```python
from build123d import *

# Parameters (mm, degrees)
F1_DEPTH  = 200
F2_R      = 15.75
F2_R_2    = 8.75
F3_DEPTH  = 20
F4_DEPTH  = 40.001
F6_DEPTH  = 89
F5_R      = 50
F7_DEPTH  = 221
F8_D      = 12.1
F9_W      = 50
F9_H      = 60
F10_DEPTH = 50
F12_DEPTH = 125.001
F13_R     = 10
F14_SIZE  = 10
F15_SIZE  = 5
F16_SIZE  = 10
F20_D     = 12.1


with BuildPart() as f1:
    # F0 (on Front) → F1 (new body)
    with BuildSketch(Plane.XZ):
        Polygon((-300, 0), (0, 0), (0, 40), (-260, 40), (-260, 300), (-300, 300), align=None)
    extrude(amount=-F1_DEPTH)

    # F2 (on face) → F3 (cut)
    with BuildSketch(Plane.XY.offset(40)):
        with Locations((-160, 160)):
            Circle(F2_R)
        with Locations((-160, 160)):
            Circle(F2_R_2, mode=Mode.SUBTRACT)
        with Locations((-160, 40)):
            Circle(F2_R)
        with Locations((-160, 40)):
            Circle(F2_R_2, mode=Mode.SUBTRACT)
        with BuildLine():
            ThreePointArc((-24.25, 40), (-28.8630681963, 51.1369318037), (-40, 55.75))
            ThreePointArc((-40, 55.75), (-51.1369318037, 28.8630681963), (-24.25, 40))
        make_face()
        with BuildLine():
            ThreePointArc((-31.25, 40), (-46.1871843354, 33.8128156646), (-40, 48.75))
            ThreePointArc((-40, 48.75), (-33.8128156646, 46.1871843354), (-31.25, 40))
        make_face(mode=Mode.SUBTRACT)
        with BuildLine():
            ThreePointArc((-24.25, 160), (-51.1369318037, 171.1369318037), (-40, 144.25))
            ThreePointArc((-40, 144.25), (-28.8630681963, 148.8630681963), (-24.25, 160))
        make_face()
        with BuildLine():
            ThreePointArc((-31.25, 160), (-33.8128156646, 153.8128156646), (-40, 151.25))
            ThreePointArc((-40, 151.25), (-46.1871843354, 166.1871843354), (-31.25, 160))
        make_face(mode=Mode.SUBTRACT)
    extrude(amount=-F3_DEPTH, mode=Mode.SUBTRACT)

    # F4 (cut, through all): faces of the model
    f4_faces = [f1.faces().sort_by_distance(p)[0] for p in [
        (-160, 160, 40),
        (-40, 160, 40),
        (-40, 40, 40),
        (-160, 40, 40),
    ]]
    extrude(f4_faces, amount=-F4_DEPTH, mode=Mode.SUBTRACT)

    # F5 (on face) → F6 (cut)
    with BuildSketch(Plane.YZ.offset(-260)):
        with BuildLine():
            ThreePointArc((0, 200), (29.2893218813, 270.7106781187), (100, 300))
            Line((100, 300), (0, 300))
            Line((0, 300), (0, 200))
        make_face()
        with BuildLine():
            ThreePointArc((100, 300), (170.7106781187, 270.7106781187), (200, 200))
            Line((200, 200), (200, 300))
            Line((200, 300), (100, 300))
        make_face()
    extrude(amount=-F6_DEPTH, mode=Mode.SUBTRACT)

    # F5 (on face) → F7 (cut)
    with BuildSketch(Plane.YZ.offset(-260)):
        with Locations((100, 200)):
            Circle(F5_R)
    extrude(amount=-F7_DEPTH, mode=Mode.SUBTRACT)

    # F8 (through all)
    with Locations(Plane.YZ.offset(-260)):
        with Locations((28, 200), (100, 272), (172, 200), (100, 128)):
            Hole(F8_D / 2)

    # F9 (on face) → F10 (join)
    with BuildSketch(Plane.YZ.offset(-260)):
        with Locations((100, 70)):
            Rectangle(F9_W, F9_H)
    extrude(amount=F10_DEPTH)

    # F11 (on face) → F12 (cut, through all)
    with BuildSketch(Plane.XZ.offset(-75)):
        Polygon((-210, 100), (-260, 100), (-210, 40), align=None)
    extrude(amount=-F12_DEPTH, mode=Mode.SUBTRACT)

    # F13
    f13_edges = [f1.edges().sort_by_distance(p)[0] for p in [
        (-260, 37.5, 40),
        (-260, 162.5, 40),
    ]]
    fillet(f13_edges, radius=F13_R)

    # F14
    f14_edges = [f1.edges().sort_by_distance(p)[0] for p in [
        (0, 0, 20),
        (0, 200, 20),
    ]]
    chamfer(f14_edges, length=F14_SIZE)

    # F15
    f15_edges = [f1.edges().sort_by_distance(p)[0] for p in [
        (-260, 50, 200),
        (-300, 50, 200),
    ]]
    chamfer(f15_edges, length=F15_SIZE)

    # F16
    f16_edges = [f1.edges().sort_by_distance(p)[0] for p in [
        (-300, 100, 0),
    ]]
    chamfer(f16_edges, length=F16_SIZE)

    # F20 (through all)
    with Locations(Plane(origin=(0, -120.7106781187, 120.7106781187), x_dir=(1, 0, 0), z_dir=(0, -0.7071067812, 0.7071067812))):
        with Locations((-280, 212.132034356)):
            Hole(F20_D / 2)


solid = f1.part
```
Verification items for the finished model (mm, model axes). A direction names the side the tool comes from. Coordinates: 2 decimals unless noted, no trailing zeros. Loops run counter-clockwise (first coordinate to the right, second up) from the corner with the lowest first, then second, coordinate; pieces in that order, holes last. Notation, with made-up numbers: (-17, 43) -> (0, 43) arc R18 ccw to (0, 48) -> close; hole circle Ø3 at (78, 21.5). An arc over 180 degrees is marked (long way). Put each result on its own line as item: value.
1. Section check B-B, the plane z = 25. Record the boundary of the cut face in (x, y).
Result set:
outline: (-300, 0) -> (-10, 0) -> (0, 10) -> (0, 190) -> (-10, 200) -> (-300, 200) -> close; hole circle Ø31.5 at (-160, 40); hole circle Ø31.5 at (-160, 160); hole circle Ø31.5 at (-40, 40); hole circle Ø31.5 at (-40, 160)
2. Section check A-A, the plane x = -160. Record the boundary of the cut face in (y, z), then the cut area to 3 significant figures.
Result set:
outline: (0, 0) -> (31.25, 0) -> (31.25, 20) -> (24.25, 20) -> (24.25, 40) -> (0, 40) -> close; (48.75, 0) -> (151.25, 0) -> (151.25, 20) -> (144.25, 20) -> (144.25, 40) -> (55.75, 40) -> (55.75, 20) -> (48.75, 20) -> close; (168.75, 0) -> (200, 0) -> (200, 40) -> (175.75, 40) -> (175.75, 20) -> (168.75, 20) -> close
area: 6,040 mm^2
3. Thickness scan on line 1 (Z direction, x = -282, y = 100); line 2 (Z direction, x = -93.5, y = 146); line 3 (X direction, y = 152.5, z = 240.5). Record the ranges inside material, lowest first.
Result set:
line 1: z = 0 to 121.95, 134.05 to 150, 250 to 265.95, 278.05 to 300
line 2: z = 0 to 40
line 3: x = -300 to -260
4. Mould release check, pull along X, two halves, no side actions. Record for faces 6 (the face through (-273.956, 47.533, 252.843)), 7 (the face through (-5, 195, 20)), 8 (the face through (-209, 0, 34)), 9 (the face through (-300, 76, 125)): pulls with the +X half, pulls with the -X half, needs draft (parallel to the pull), parting line crosses it, or undercut.
Result set:
face 6: undercut
face 7: pulls with the +X half
face 8: needs draft
face 9: pulls with the -X half
5. Section check C-C, the plane z = 79. Record the boundary of the cut face in (x, y).
Result set:
outline: (-300, 0) -> (-260, 0) -> (-260, 75) -> (-242.5, 75) -> (-242.5, 125) -> (-260, 125) -> (-260, 200) -> (-300, 200) -> close
6. Tool access check on faces 1 (the face through (-256.99, 38.02, 42.85)), 2 (the face through (-144.977, 44.731, 30.14)), 3 (the face through (-151.917, 36.649, 10.14)), 4 (the face through (-280.28, 166.23, 201.82)), 5 (the face through (-256.99, 163.02, 42.85)). Record the directions out of +Z, -Z, +X, -X, +Y, -Y that give a thin tool (end or side, any length) a straight path to the whole face; none if there is none.
Result set:
face 1: +Z, +X, -Y
face 2: +Z
face 3: +Z, -Z
face 4: +X, -X
face 5: +Z, +X, +Y
7. Gauge pin test, flat ends, axial feed: P1, Ø5, axis at x = -176.5, y = 112, coming from the +Z side; P2, Ø25, axis at x = -40, y = 40, coming from the +Z side; P3, Ø6, axis at y = 37, z = 53.5, coming from the +X side. Record the tip position at first contact, or that the pin passes through.
Result set:
P1: stops at z = 40
P2: stops at z = 20
P3: stops at x = -260
8. Section check D-D, the plane z = 128. Give the number of separate pieces and of enclosed holes in the cut face, then the cut area to 3 significant figures.
Result set:
separate pieces: 2
enclosed holes: 1
area: 7,350 mm^2
